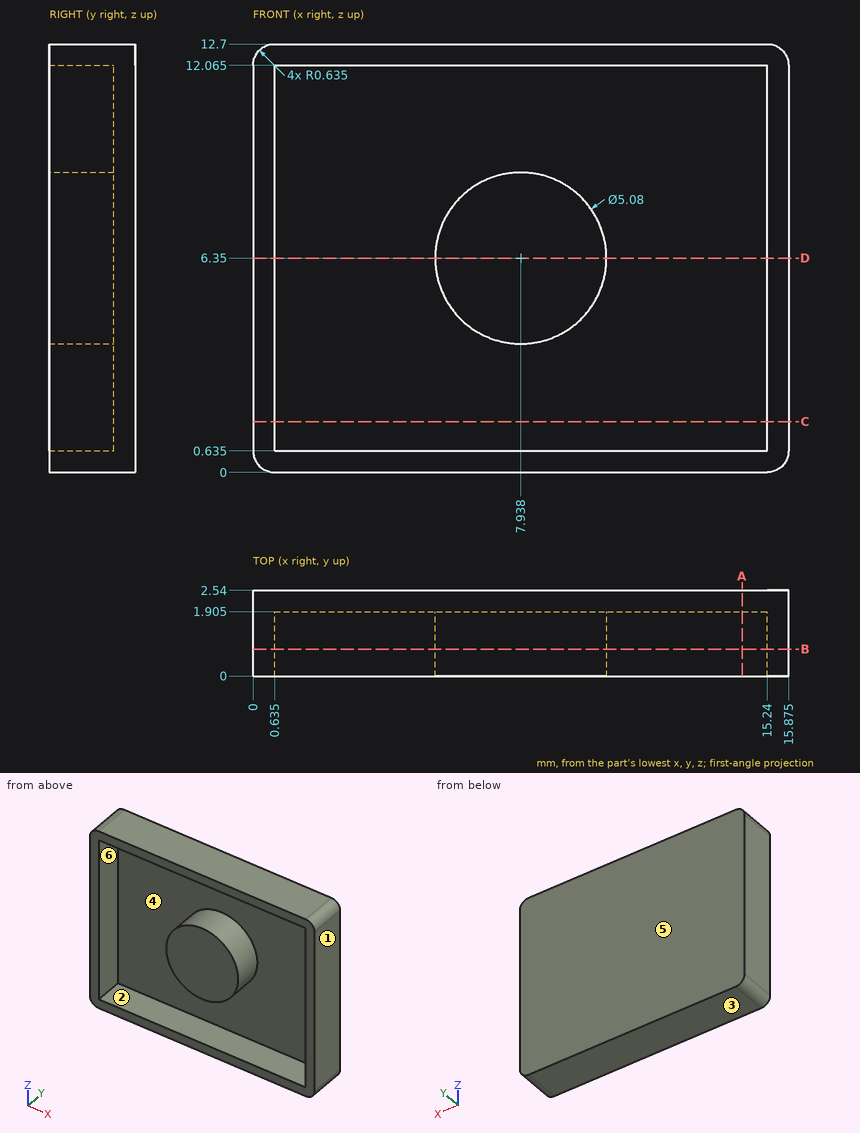
Here's the drawing with two shaded views (mm, measured from the low corner). I have some questions. A direction names the side the tool comes from. Round coordinates to 2 decimals unless told otherwise and drop trailing zeros. Order: outer loops, then holes, each group sorted by start corner. A loop starts at its lowest first (then second) coordinate and runs counter-clockwise, first axis right, second up. Notation, with made-up numbers: (42, 84.25) -> (76, 84.25) arc R9 cw to (76, 93.25) -> close; hole circle Ø3 at (38, 81). An arc over 180 degrees is marked (long way). Write each question's results on one line, items separated by ' | '. Start each with the question number.
Item 1: Please list where these lines run through material, in increasing order: L1, parallel to X at y = 1.5, z = 1.75 (1 decimal); L2, parallel to Z at x = 6.5, y = 0.65 (1 decimal); L3, parallel to X at y = 1.25, z = 8 (1 decimal).
Item 2: If we section it at A-A, the plane x = 14.5: Write out the boundary of the cut face in (y, z) (1 decimal).
Item 3: If we section it at C-C, the plane z = 1.5: Write out the boundary of the cut face in (x, y) (1 decimal), then the cut area to 3 significant figures.
Item 4: Which directions (+Z, -Z, +X, -X, +Y, -Y) give clear straight access to the entire face, cutting with the end or side of a thin tool? Please do the marked faces 5 and 6.
Item 5: Thinking about a two-plate mould opening in Z: for the marked faces 1, 2, 3 and 4, which applies, +Z half, -Z half, draft (parallel to the pull), parting line (faces both ways), or undercut?
Item 6: If we section it at B-B, the plane y = 0.8: State how many separate pieces and enclosed holes the cut face has.
Item 7: If we section it at D-D, the plane z = 6.35: Write out the boundary of the cut face in (x, y) (1 decimal).
Results:
1) L1: x = 0 to 0.6, 15.2 to 15.9 | L2: z = 0 to 0.6, 4.3 to 8.4, 12.1 to 12.7 | L3: x = 0 to 0.6, 6 to 9.9, 15.2 to 15.9
2) outline: (0, 0) -> (2.5, 0) -> (2.5, 12.7) -> (0, 12.7) -> (0, 12.1) -> (1.9, 12.1) -> (1.9, 0.6) -> (0, 0.6) -> close
3) outline: (0, 0) -> (0.6, 0) -> (0.6, 1.9) -> (15.2, 1.9) -> (15.2, 0) -> (15.9, 0) -> (15.9, 2.5) -> (0, 2.5) -> close | area: 12.5 mm2
4) face 5: +Z, -Z, +X, -X, +Y | face 6: -Y
5) face 1: draft | face 2: undercut | face 3: -Z half | face 4: undercut
6) separate pieces: 2 | enclosed holes: 1
7) outline: (0, 0) -> (0.6, 0) -> (0.6, 1.9) -> (5.4, 1.9) -> (5.4, 0) -> (10.5, 0) -> (10.5, 1.9) -> (15.2, 1.9) -> (15.2, 0) -> (15.9, 0) -> (15.9, 2.5) -> (0, 2.5) -> close
